Autodesk Inventor part; units mm, degrees
ref_plane "1_XY" through (27.0002, 0, 0) normal (1, 0, 0) x (0, 0, -1)
ref_plane "1_YZ" through (27.0002, 0, 0) normal (0, 0, -1) x (0, 1, 0)
ref_plane "1_ZX" through (27.0002, 0, 0) normal (0, 1, 0) x (1, 0, 0)
sketch "Sketch_8" plane through (0, 0, 0) normal (0, 0, 1) x (1, 0, 0)
  line L0 (24.6126, 0) -> (0, 0)
  line L1 (0, 0) -> (0, 8.9091)
  line L2 (0, 8.9091) -> (0.762, 9.671)
  line L3 (0.762, 9.671) -> (4.0386, 9.671)
  line L4 (4.0386, 9.671) -> (4.8006, 8.9091)
  line L5 (4.8006, 8.9091) -> (5.5626, 8.9091)
  line L6 (5.5626, 8.9091) -> (5.5626, 10.3759)
  line L7 (5.5626, 10.3759) -> (8.7363, 10.3759)
  line L8 (8.7363, 10.3759) -> (9.3142, 10.9537)
  line L9 (9.3142, 10.9537) -> (23.8506, 10.9537)
  line L10 (23.8506, 10.9537) -> (24.6126, 10.1917)
  line L11 (24.6126, 10.1917) -> (24.6126, 0)
  line L12 (24.6126, 0) -> (0, 0)
revolve "Revolution1" add sketch "Sketch_8" angle 360 about axis through (24.6126, 0, 0) along (1, 0, 0)
sketch "Sketch_15" plane through (0, 0, 0) normal (0, 0, 1) x (1, 0, 0)
  line L0 (40.4876, 0) -> (24.6126, 0)
  line L1 (24.6126, 0) -> (24.6126, 7.9057)
  line L2 (24.6126, 7.9057) -> (27.0002, 7.9057)
  line L3 (27.0002, 7.9057) -> (27.0002, 7.7279)
  arc A0 (27.0002, 7.7279) -> (27.8892, 6.839) centre (27.8892, 7.728) ccw
  line L4 (27.8892, 6.839) -> (29.1719, 6.839)
  arc A1 (29.1719, 6.839) -> (29.7706, 7.0708) centre (29.1719, 7.7279) ccw
  line L5 (29.7706, 7.0708) -> (29.8005, 7.098)
  line L6 (29.8005, 7.098) -> (30.64, 7.9375)
  line L7 (30.64, 7.9375) -> (39.6481, 7.9375)
  line L8 (39.6481, 7.9375) -> (40.4876, 7.098)
  line L9 (40.4876, 7.098) -> (40.4876, 0)
  line L10 (40.4876, 0) -> (24.6126, 0)
revolve "Revolution2" add sketch "Sketch_15" angle 360 about axis through (40.4876, 0, 0) along (1, 0, 0)
thread "Thread1"
sketch "Sketch_70" plane through (40.4876, 0, 0) normal (1, 0, 0) x (0, 0, -1)
  line L0 (-43.815, -21.9075) -> (43.815, -21.9075)
  line L1 (43.815, -21.9075) -> (43.815, 21.9075)
  line L2 (43.815, 21.9075) -> (-43.815, 21.9075)
  line L3 (-43.815, 21.9075) -> (-43.815, -21.9075)
  line L4 (-21.9075, -4.7308) -> (21.9075, -4.7308)
  line L5 (21.9075, -4.7308) -> (21.9075, 4.7308)
  line L6 (21.9075, 4.7308) -> (-21.9075, 4.7308)
  line L7 (-21.9075, 4.7308) -> (-21.9075, -4.7308)
extrude "Extrusion1" cut sketch "Sketch_70" against normal blind 15.875
sketch "Sketch4" plane through (0, 0, 0) normal (-1, 0, 0) x (0, 0, 1)
  point P0 (0, 0)
hole "Hole1" at (0, 0, 0) direction (1, 0, 0) diameter 7.9248 depth 23.5814 tip angle 120
sketch "Sketch_47" plane through (0, 0, 0) normal (0, 0, 1) x (1, 0, 0)
  line L0 (17.4752, 0) -> (17.4752, 10.9537)
  line L1 (17.4752, 10.9537) -> (22.9299, 10.9537)
  line L2 (22.9299, 10.9537) -> (22.2949, 10.3187)
  line L3 (22.2949, 10.3187) -> (22.04, 2.1565)
  line L4 (22.04, 2.1565) -> (22.04, 0)
  line L5 (22.04, 0) -> (17.4752, 0)
  line L6 (17.4752, 0) -> (17.4752, 10.9537)
revolve "Revolution3" cut sketch "Sketch_47" angle 360 about axis through (17.4752, 0, 0) along (0, -1, 0)
thread "Thread2"
sketch "Sketch_24" plane through (0, 0, 0) normal (0, 0, 1) x (1, 0, 0)
  line L0 (5.5626, 0) -> (4.8006, 0)
  line L1 (4.4955, 10.3759) -> (4.4955, 10.2917)
  line L2 (4.4955, 10.2917) -> (5.4401, 9.3472)
  arc A0 (5.4401, 9.1676) -> (5.4401, 9.3472) centre (5.3503, 9.2574) ccw
  line L3 (5.4401, 9.1676) -> (5.1816, 8.9091)
  line L4 (5.1816, 8.9091) -> (4.8006, 8.9091)
  line L5 (4.8006, 8.9091) -> (4.8006, 8.655)
  line L6 (4.8006, 8.655) -> (5.5626, 8.655)
  line L7 (5.5626, 8.655) -> (5.5626, 9.512)
  line L8 (5.5626, 9.512) -> (4.6987, 10.3759)
  line L9 (4.6987, 10.3759) -> (4.4955, 10.3759)
revolve "Revolution4" add sketch "Sketch_24" angle 360 about axis through (5.5626, 0, 0) along (1, 0, 0)
sketch "Sketch_43" plane through (0, 0, 0) normal (0, 1, 0) x (-1, 0, 0)
  circle A0 centre (-33.3248, 0) radius 4.3879
extrude "Extrusion2" cut sketch "Sketch_43" along normal mid plane 14.1922
ref_plane "1_XY" through (27.0002, 0, 0) normal (1, 0, 0) x (0, 0, -1)
ref_plane "1_YZ" through (27.0002, 0, 0) normal (0, 0, -1) x (0, 1, 0)
ref_plane "1_ZX" through (27.0002, 0, 0) normal (0, 1, 0) x (1, 0, 0)
ref_plane "c1_XY" through (24.6126, 7.9057, 0) normal (0, 0, 1) x (1, 0, 0)
ref_plane "c1_YZ" through (24.6126, 7.9057, 0) normal (1, 0, 0) x (0, 1, 0)
ref_plane "c1_ZX" through (24.6126, 7.9057, 0) normal (0, 1, 0) x (0, 0, 1)
ref_plane "c2_XY" through (24.6126, -7.9057, 0) normal (0, 0, 1) x (1, 0, 0)
ref_plane "c2_YZ" through (24.6126, -7.9057, 0) normal (1, 0, 0) x (0, 1, 0)
ref_plane "c2_ZX" through (24.6126, -7.9057, 0) normal (0, 1, 0) x (0, 0, 1)
ref_plane "cc1_XY" through (24.6126, 0, 0) normal (0, 0, 1) x (1, 0, 0)
ref_plane "cc1_YZ" through (24.6126, 0, 0) normal (1, 0, 0) x (0, 1, 0)
ref_plane "cc1_ZX" through (24.6126, 0, 0) normal (0, 1, 0) x (0, 0, 1)
ref_plane "cc2_XY" through (27.0002, 0, 0) normal (0, 0, 1) x (1, 0, 0)
ref_plane "cc2_YZ" through (27.0002, 0, 0) normal (1, 0, 0) x (0, 1, 0)
ref_plane "cc2_ZX" through (27.0002, 0, 0) normal (0, 1, 0) x (0, 0, 1)
ref_plane "lovra1_XY" through (35.7124, 0, 0) normal (1, 0, 0) x (0, 0, -1)
ref_plane "lovra1_YZ" through (35.7124, 0, 0) normal (0, 0, -1) x (0, 1, 0)
ref_plane "lovra1_ZX" through (35.7124, 0, 0) normal (0, 1, 0) x (1, 0, 0)
ref_plane "lovra2_XY" through (35.7124, 7.874, 0) normal (1, 0, 0) x (0, 0, -1)
ref_plane "lovra2_YZ" through (35.7124, 7.874, 0) normal (0, 0, -1) x (0, 1, 0)
ref_plane "lovra2_ZX" through (35.7124, 7.874, 0) normal (0, 1, 0) x (1, 0, 0)
ref_plane "lovra21_XY" through (0, 0, 5.2705) normal (1, 0, 0) x (0, 0, -1)
ref_plane "lovra21_YZ" through (0, 0, 5.2705) normal (0, 0, -1) x (0, 1, 0)
ref_plane "lovra21_ZX" through (0, 0, 5.2705) normal (0, 1, 0) x (1, 0, 0)
ref_plane "lovra22_XY" through (0, 0, -5.2705) normal (1, 0, 0) x (0, 0, -1)
ref_plane "lovra22_YZ" through (0, 0, -5.2705) normal (0, 0, -1) x (0, 1, 0)
ref_plane "lovra22_ZX" through (0, 0, -5.2705) normal (0, 1, 0) x (1, 0, 0)
ref_plane "lovra3_XY" through (35.7124, -7.874, 0) normal (1, 0, 0) x (0, 0, -1)
ref_plane "lovra3_YZ" through (35.7124, -7.874, 0) normal (0, 0, -1) x (0, 1, 0)
ref_plane "lovra3_ZX" through (35.7124, -7.874, 0) normal (0, 1, 0) x (1, 0, 0)
ref_plane "olen_XY" through (33.3248, 0, 0) normal (1, 0, 0) x (0, 0, -1)
ref_plane "olen_YZ" through (33.3248, 0, 0) normal (0, 0, -1) x (0, 1, 0)
ref_plane "olen_ZX" through (33.3248, 0, 0) normal (0, 1, 0) x (1, 0, 0)
ref_plane "p1_XY" through (40.4876, 0, 4.7308) normal (1, 0, 0) x (0, 0, -1)
ref_plane "p1_YZ" through (40.4876, 0, 4.7308) normal (0, 0, -1) x (0, 1, 0)
ref_plane "p1_ZX" through (40.4876, 0, 4.7308) normal (0, 1, 0) x (1, 0, 0)
ref_plane "p2_XY" through (40.4876, 0, -4.7308) normal (1, 0, 0) x (0, 0, -1)
ref_plane "p2_YZ" through (40.4876, 0, -4.7308) normal (0, 0, -1) x (0, 1, 0)
ref_plane "p2_ZX" through (40.4876, 0, -4.7308) normal (0, 1, 0) x (1, 0, 0)
ref_plane "port_XY" through (17.4752, 0, 0) normal (0, 0, 1) x (1, 0, 0)
ref_plane "port_YZ" through (17.4752, 0, 0) normal (1, 0, 0) x (0, 1, 0)
ref_plane "port_ZX" through (17.4752, 0, 0) normal (0, 1, 0) x (0, 0, 1)
ref_plane "port2_XY" through (40.4876, 0, 0) normal (1, 0, 0) x (0, 0, -1)
ref_plane "port2_YZ" through (40.4876, 0, 0) normal (0, 0, -1) x (0, 1, 0)
ref_plane "port2_ZX" through (40.4876, 0, 0) normal (0, 1, 0) x (1, 0, 0)
ref_plane "thd1_XY" through (40.4876, 0, 7.9375) normal (1, 0, 0) x (0, 0, -1)
ref_plane "thd1_YZ" through (40.4876, 0, 7.9375) normal (0, 0, -1) x (0, 1, 0)
ref_plane "thd1_ZX" through (40.4876, 0, 7.9375) normal (0, 1, 0) x (1, 0, 0)
ref_plane "thd2_XY" through (40.4876, 0, -7.9375) normal (1, 0, 0) x (0, 0, -1)
ref_plane "thd2_YZ" through (40.4876, 0, -7.9375) normal (0, 0, -1) x (0, 1, 0)
ref_plane "thd2_ZX" through (40.4876, 0, -7.9375) normal (0, 1, 0) x (1, 0, 0)
ref_plane "to_mounting_bracket_XY" through (24.6126, 0, 0) normal (1, 0, 0) x (0, 0, -1)
ref_plane "to_mounting_bracket_YZ" through (24.6126, 0, 0) normal (0, 0, -1) x (0, 1, 0)
ref_plane "to_mounting_bracket_ZX" through (24.6126, 0, 0) normal (0, 1, 0) x (1, 0, 0)
ref_plane "to_nut_XY" through (27.0002, 0, 0) normal (1, 0, 0) x (0, 0, -1)
ref_plane "to_nut_YZ" through (27.0002, 0, 0) normal (0, 0, -1) x (0, 1, 0)
ref_plane "to_nut_ZX" through (27.0002, 0, 0) normal (0, 1, 0) x (1, 0, 0)
ref_plane "to_pin_XY" through (33.3248, 0, 0) normal (0, 1, 0) x (1, 0, 0)
ref_plane "to_pin_YZ" through (33.3248, 0, 0) normal (1, 0, 0) x (0, 0, -1)
ref_plane "to_pin_ZX" through (33.3248, 0, 0) normal (0, 0, -1) x (0, 1, 0)
ref_plane "to_pin_1_XY" through (33.3248, 0, 0) normal (0, 0, 1) x (1, 0, 0)
ref_plane "to_pin_1_YZ" through (33.3248, 0, 0) normal (1, 0, 0) x (0, 1, 0)
ref_plane "to_pin_1_ZX" through (33.3248, 0, 0) normal (0, 1, 0) x (0, 0, 1)
ref_plane "to_pin_r_XY" through (33.3248, 0, 0) normal (0, 0, 1) x (1, 0, 0)
ref_plane "to_pin_r_YZ" through (33.3248, 0, 0) normal (1, 0, 0) x (0, 1, 0)
ref_plane "to_pin_r_ZX" through (33.3248, 0, 0) normal (0, 1, 0) x (0, 0, 1)
ref_plane "to_screw_XY" through (17.4752, 2.032, -6.0452) normal (0, 1, 0) x (1, 0, 0)
ref_plane "to_screw_YZ" through (17.4752, 2.032, -6.0452) normal (1, 0, 0) x (0, 0, -1)
ref_plane "to_screw_ZX" through (17.4752, 2.032, -6.0452) normal (0, 0, -1) x (0, 1, 0)
ref_plane "to_tube_XY" through (4.8006, 0, 0) normal (1, 0, 0) x (0, 0, -1)
ref_plane "to_tube_YZ" through (4.8006, 0, 0) normal (0, 0, -1) x (0, 1, 0)
ref_plane "to_tube_ZX" through (4.8006, 0, 0) normal (0, 1, 0) x (1, 0, 0)
properties part number "04P0Y000_rear_head"
Here's how the part is built. I have some questions about the finished solid (model axes, mm). A direction names the side the tool comes from. Coordinates: 2 decimals unless noted, no trailing zeros. Write each loop counter-clockwise with the first axis right and the second up, starting at its lowest first coordinate (ties: lowest second). Pieces come first, ordered by that corner, then holes. Notation, with made-up numbers: (73.25, -9.5) - (99.25, -9.5) arc R22 ccw to (99.25, 0.5) - close; hole circle Ø10 at (-2, 27). An arc over 180 degrees is marked (long way). Use one line per item in the form item = value.
1) Suppose I cut it at A-A, the plane x = 35.5. Write out the boundary of the cut face in (y, z) (1 decimal), plus the area to 3 significant figures.
Solved:
outline = (-4.7, -6.4) arc R7.9 ccw to (4.7, -6.4) - (4.7, -3.8) - (-4.7, -3.8) - close; (-4.7, 3.8) - (4.7, 3.8) - (4.7, 6.4) arc R7.9 ccw to (-4.7, 6.4) - close
area = 68.7 mm2
2) Thinking about a two-plate mould opening in X: for faces 1 (the flat face through (29, 4.731, -2)), 2 (the conical face through (19.999, 6.295, -3.958)), 3 (the conical face through (40.342, -0.074, 7.243)), 4 (the cylindrical face through (28.54, 0.07, 6.84)), which applies, released by +X, released by -X, zero draft, split by the parting line, or undercut?
Solved:
face_1 = zero draft
face_2 = undercut
face_3 = released by +X
face_4 = undercut
3) Suppose I cut it at B-B, the plane x = 11. Write out the boundary of the cut face in (y, z), plus the area to 3 significant figures.
Solved:
outline = circle Ø21.91 at (0, 0); hole circle Ø7.92 at (0, 0)
area = 328 mm2
4) Suppose I cut it at C-C, the plane z = 0.5. Give the number of separate pieces and of enclosed holes in the cut face, plus the area to 3 significant figures.
Solved:
separate_pieces = 3
enclosed_holes = 0
area = 326 mm2
5) On a 3-axis mill with a long thin cutter (end or side, diameter ignored), from which of +Z, -Z, +X, -X, +Y, -Y can I reach the whole of each face in a straight line? I mean faces 5 (the flat face through (40.488, 0, 0)), 6 (the cylindrical face through (7.172, -10.366, 0.456)), 7 (the conical face through (29.946, -0.074, -7.243)). Say none if no direction works.
Solved:
face_5 = +Z, -Z, +X, +Y, -Y
face_6 = -X
face_7 = -Z
6) I'm going to push flat-ended pins straight in: P1, Ø8, axis at x = 33.32, z = 0, coming from the +Y side (3 decimals); P2, Ø6.5, axis at y = 0, z = 0, coming from the -X side; P3, Ø6.5, axis at x = 29.5, z = 1, coming from the +Y side; P4, Ø3, axis at x = 25, z = -2, coming from the +Y side. Where does each tip first touch, or does it pass through?
Solved:
P1 = through
P2 = 23.99
P3 = 4.73
P4 = 10.9
7) I need wall thicknesses on line 1 (Z direction, x = 7.5, y = 0); line 2 (Z direction, x = 4, y = 0.25); line 3 (X direction, y = 3.5, z = 2.75). Which ranges of each line are inside material? Lowest first, please.
Solved:
line_1 = -10.38 to -3.96, 3.96 to 10.38
line_2 = -9.67 to -3.95, 3.95 to 9.67
line_3 = 0 to 13.78, 21.17 to 29.91, 36.74 to 40.49
